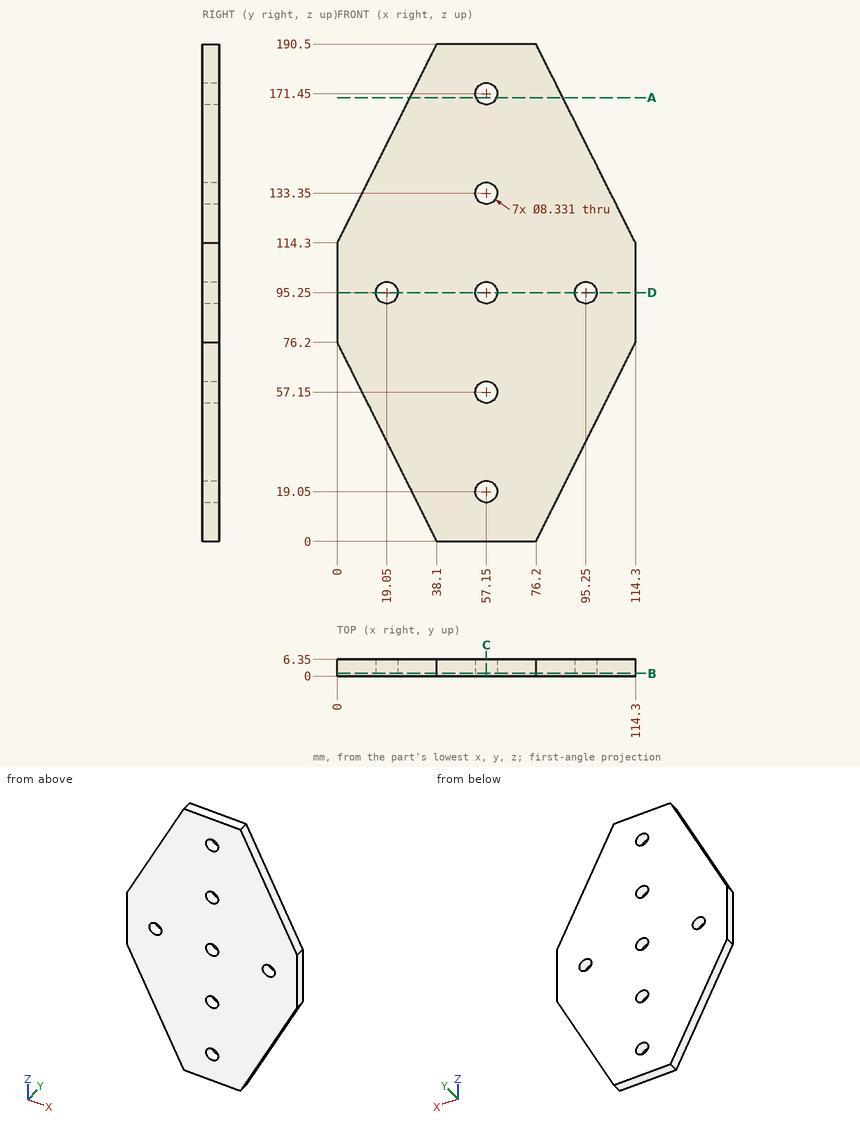
The drawing under review shows one solid part. Ordinate dimensions are in mm from its lowest x, y, z. Round coordinates to 2 decimals unless told otherwise and drop trailing zeros. Loops run counter-clockwise (first coordinate to the right, second up) from the corner with the lowest first, then second, coordinate; pieces in that order, holes last. Notation, with made-up numbers: (4, 19.25) - (24, 19.25) arc R21 ccw to (24, 36.25) - close; hole circle Ø4 at (-10, -37). An arc over 180 degrees is marked (long way). Use one line per item in the form item = value.
Item 1: For line 1 (X direction, y = 2.25, z = 95.25); line 2 (Z direction, x = 59, y = 1); line 3 (X direction, y = 2, z = 55), list the stretches that pass through material, from the lowest coordinate up.
Answers:
line_1 = 0 to 14.88, 23.22 to 52.98, 61.32 to 91.08, 99.42 to 114.3
line_2 = 0 to 15.32, 22.78 to 53.42, 60.88 to 91.52, 98.98 to 129.62, 137.08 to 167.72, 175.18 to 190.5
line_3 = 10.6 to 53.58, 60.72 to 103.7
Item 2: Consider section C-C on x = 57.15. Write out the cut boundary in (y, z).
Answers:
outline = (0, 0) - (6.35, 0) - (6.35, 14.88) - (0, 14.88) - close; (0, 23.22) - (6.35, 23.22) - (6.35, 52.98) - (0, 52.98) - close; (0, 61.32) - (6.35, 61.32) - (6.35, 91.08) - (0, 91.08) - close; (0, 99.42) - (6.35, 99.42) - (6.35, 129.18) - (0, 129.18) - close; (0, 137.52) - (6.35, 137.52) - (6.35, 167.28) - (0, 167.28) - close; (0, 175.62) - (6.35, 175.62) - (6.35, 190.5) - (0, 190.5) - close
Item 3: Consider section D-D on z = 95.25. Write out the cut boundary in (x, y), then the cut area to 3 significant figures.
Answers:
outline = (0, 0) - (14.88, 0) - (14.88, 6.35) - (0, 6.35) - close; (23.22, 0) - (52.98, 0) - (52.98, 6.35) - (23.22, 6.35) - close; (61.32, 0) - (91.08, 0) - (91.08, 6.35) - (61.32, 6.35) - close; (99.42, 0) - (114.3, 0) - (114.3, 6.35) - (99.42, 6.35) - close
area = 567 mm^2
Item 4: Clearance check with flat-ended pins moving along their axes: P1, Ø11, axis at x = 57.15, z = 57.15, coming from the +Y side; P2, Ø7.5, axis at x = 19.05, z = 95.25, coming from the -Y side; P3, Ø2, axis at x = 79, y = 5, coming from the +Z side. State where each tip first meets the part, or that it passes through.
Answers:
P1 = 6.35
P2 = through
P3 = 186.9
Item 5: Consider section A-A on z = 170. Write out the cut boundary in (x, y) (3 decimals).
Answers:
outline = (27.85, 0) - (53.245, 0) - (53.245, 6.35) - (27.85, 6.35) - close; (61.055, 0) - (86.45, 0) - (86.45, 6.35) - (61.055, 6.35) - close
Item 6: Consider section B-B on y = 1. Write out the cut boundary in (x, z), then the cut area to 3 significant figures.
Answers:
outline = (0, 76.2) - (38.1, 0) - (76.2, 0) - (114.3, 76.2) - (114.3, 114.3) - (76.2, 190.5) - (38.1, 190.5) - (0, 114.3) - close; hole circle Ø8.33 at (19.05, 95.25); hole circle Ø8.33 at (57.15, 19.05); hole circle Ø8.33 at (57.15, 57.15); hole circle Ø8.33 at (57.15, 95.25); hole circle Ø8.33 at (57.15, 133.35); hole circle Ø8.33 at (57.15, 171.45); hole circle Ø8.33 at (95.25, 95.25)
area = 15,600 mm^2
